The model under review builds one solid part; all positions refer to its coordinate system, in mm. Round coordinates to 2 decimals unless told otherwise and drop trailing zeros. Answer as a JSON object with one key per item and string values. Group by question number.
1. To check wall thickness, follow probe 1 along Y at (x, z) = (0, -487); probe 2 along Y at (x, z) = (-5, -238.5); probe 3 along Y at (x, z) = (-7.5, -543). State the ranges of each line that lie inside material, in increasing order. Write a range as [from, to].
2. Add section A-A on z = -559. Give the number of separate pieces and of enclosed holes in the cut face, and give its area (3 significant figures).
3. Clearance check with flat-ended pins moving along their axes: P1, Ø2.5, axis at x = 1.5, z = -398.5, coming from the +Y side; P2, Ø1.1, axis at x = 1.5, z = -214.5, coming from the -Y side. State where each tip first meets the part, or that it passes through.
```python
from build123d import *

# Parameters (mm, degrees)
SKETCH1_R           = 2.5
BOSS_EXTRUDE1_DEPTH = 550


with BuildPart() as part:
    # Sketch1 → Boss-Extrude1 (new body)
    with BuildSketch(Plane(origin=(0, 0, -600), x_dir=(-1, 0, 0), z_dir=(0, 0, -1))):
        with BuildLine():
            Line((10, -7), (10, 7))
            Line((10, 7), (8, 7))
            Line((8, 7), (8, 4))
            Line((8, 4), (7.060660172, 4))
            Line((7.060660172, 4), (4, 7.060660172))
            Line((4, 7.060660172), (4, 7.5))
            Line((4, 7.5), (3.750976592, 8.781114371))
            Line((3.750976592, 8.781114371), (3.933012702, 9.096410162))
            ThreePointArc((3.933012702, 9.096410162), (4, 9.346410162), (3.933012702, 9.596410162))
            Line((3.933012702, 9.596410162), (3.7, 10))
            Line((3.7, 10), (3.933012702, 10.403589838))
            ThreePointArc((3.933012702, 10.403589838), (3.982962913, 10.524180316), (4, 10.653589838))
            Line((4, 10.653589838), (4, 12.939339828))
            Line((4, 12.939339828), (7.060660172, 16))
            Line((7.060660172, 16), (8, 16))
            Line((8, 16), (8, 13))
            Line((8, 13), (10, 13))
            Line((10, 13), (10, 19))
            ThreePointArc((10, 19), (9.707106781, 19.707106781), (9, 20))
            Line((9, 20), (3, 20))
            Line((3, 20), (3, 18))
            Line((3, 18), (6, 18))
            Line((6, 18), (6, 17.060660172))
            Line((6, 17.060660172), (2.939339828, 14))
            Line((2.939339828, 14), (2.5, 14))
            Line((2.5, 14), (1.218885629, 13.750976592))
            Line((1.218885629, 13.750976592), (0.903589838, 13.933012702))
            ThreePointArc((0.903589838, 13.933012702), (0.653589838, 14), (0.403589838, 13.933012702))
            Line((0.403589838, 13.933012702), (0, 13.7))
            Line((0, 13.7), (-0.403589838, 13.933012702))
            ThreePointArc((-0.403589838, 13.933012702), (-0.524180316, 13.982962913), (-0.653589838, 14))
            Line((-0.653589838, 14), (-2.939339828, 14))
            Line((-2.939339828, 14), (-6, 17.060660172))
            Line((-6, 17.060660172), (-6, 18))
            Line((-6, 18), (-3, 18))
            Line((-3, 18), (-3, 20))
            Line((-3, 20), (-9, 20))
            ThreePointArc((-9, 20), (-9.707106781, 19.707106781), (-10, 19))
            Line((-10, 19), (-10, 13))
            Line((-10, 13), (-8, 13))
            Line((-8, 13), (-8, 16))
            Line((-8, 16), (-7.060660172, 16))
            Line((-7.060660172, 16), (-4, 12.939339828))
            Line((-4, 12.939339828), (-4, 12.5))
            Line((-4, 12.5), (-3.750976592, 11.218885629))
            Line((-3.750976592, 11.218885629), (-3.933012702, 10.903589838))
            ThreePointArc((-3.933012702, 10.903589838), (-4, 10.653589838), (-3.933012702, 10.403589838))
            Line((-3.933012702, 10.403589838), (-3.7, 10))
            Line((-3.7, 10), (-3.933012702, 9.596410162))
            ThreePointArc((-3.933012702, 9.596410162), (-3.982962913, 9.475819684), (-4, 9.346410162))
            Line((-4, 9.346410162), (-4, 7.060660172))
            Line((-4, 7.060660172), (-7.060660172, 4))
            Line((-7.060660172, 4), (-8, 4))
            Line((-8, 4), (-8, 7))
            Line((-8, 7), (-10, 7))
            Line((-10, 7), (-10, -7))
            Line((-10, -7), (-8, -7))
            Line((-8, -7), (-8, -4))
            Line((-8, -4), (-7.060660172, -4))
            Line((-7.060660172, -4), (-4, -7.060660172))
            Line((-4, -7.060660172), (-4, -9.346410162))
            ThreePointArc((-4, -9.346410162), (-3.982962913, -9.475819684), (-3.933012702, -9.596410162))
            Line((-3.933012702, -9.596410162), (-3.7, -10))
            Line((-3.7, -10), (-3.933012702, -10.403589838))
            ThreePointArc((-3.933012702, -10.403589838), (-4, -10.653589838), (-3.933012702, -10.903589838))
            Line((-3.933012702, -10.903589838), (-3.750976592, -11.218885629))
            Line((-3.750976592, -11.218885629), (-4, -12.5))
            Line((-4, -12.5), (-4, -12.939339828))
            Line((-4, -12.939339828), (-7.060660172, -16))
            Line((-7.060660172, -16), (-8, -16))
            Line((-8, -16), (-8, -13))
            Line((-8, -13), (-10, -13))
            Line((-10, -13), (-10, -19))
            ThreePointArc((-10, -19), (-9.707106781, -19.707106781), (-9, -20))
            Line((-9, -20), (-3, -20))
            Line((-3, -20), (-3, -18))
            Line((-3, -18), (-6, -18))
            Line((-6, -18), (-6, -17.060660172))
            Line((-6, -17.060660172), (-2.939339828, -14))
            Line((-2.939339828, -14), (-0.653589838, -14))
            ThreePointArc((-0.653589838, -14), (-0.524180316, -13.982962913), (-0.403589838, -13.933012702))
            Line((-0.403589838, -13.933012702), (0, -13.7))
            Line((0, -13.7), (0.403589839, -13.933012702))
            ThreePointArc((0.403589839, -13.933012702), (0.653589839, -14), (0.903589838, -13.933012702))
            Line((0.903589838, -13.933012702), (1.218885629, -13.750976592))
            Line((1.218885629, -13.750976592), (2.5, -14))
            Line((2.5, -14), (2.939339828, -14))
            Line((2.939339828, -14), (6, -17.060660172))
            Line((6, -17.060660172), (6, -18))
            Line((6, -18), (3, -18))
            Line((3, -18), (3, -20))
            Line((3, -20), (9, -20))
            ThreePointArc((9, -20), (9.707106781, -19.707106781), (10, -19))
            Line((10, -19), (10, -13))
            Line((10, -13), (8, -13))
            Line((8, -13), (8, -16))
            Line((8, -16), (7.060660172, -16))
            Line((7.060660172, -16), (4, -12.939339828))
            Line((4, -12.939339828), (4, -10.653589838))
            ThreePointArc((4, -10.653589838), (3.982962913, -10.524180316), (3.933012702, -10.403589838))
            Line((3.933012702, -10.403589838), (3.7, -10))
            Line((3.7, -10), (3.933012702, -9.596410162))
            ThreePointArc((3.933012702, -9.596410162), (4, -9.346410162), (3.933012702, -9.096410162))
            Line((3.933012702, -9.096410162), (3.750976592, -8.781114371))
            Line((3.750976592, -8.781114371), (4, -7.5))
            Line((4, -7.5), (4, -7.060660172))
            Line((4, -7.060660172), (7.060660172, -4))
            Line((7.060660172, -4), (8, -4))
            Line((8, -4), (8, -7))
            Line((8, -7), (10, -7))
        make_face()
        with Locations((0, -10)):
            Circle(SKETCH1_R, mode=Mode.SUBTRACT)
        with Locations((0, 10)):
            Circle(SKETCH1_R, mode=Mode.SUBTRACT)
        with BuildLine():
            Line((8, 1.7), (8, -1.7))
            ThreePointArc((8, -1.7), (7.912132034, -1.912132034), (7.7, -2))
            Line((7.7, -2), (7.063603897, -2))
            ThreePointArc((7.063603897, -2), (6.948798867, -2.02283614), (6.851471863, -2.087867966))
            Line((6.851471863, -2.087867966), (2.939339828, -6))
            Line((2.939339828, -6), (-2.939339828, -6))
            Line((-2.939339828, -6), (-6.851471863, -2.087867966))
            ThreePointArc((-6.851471863, -2.087867966), (-6.948798867, -2.02283614), (-7.063603897, -2))
            Line((-7.063603897, -2), (-7.7, -2))
            ThreePointArc((-7.7, -2), (-7.912132034, -1.912132034), (-8, -1.7))
            Line((-8, -1.7), (-8, 1.7))
            ThreePointArc((-8, 1.7), (-7.912132034, 1.912132034), (-7.7, 2))
            Line((-7.7, 2), (-7.063603897, 2))
            ThreePointArc((-7.063603897, 2), (-6.948798867, 2.02283614), (-6.851471863, 2.087867966))
            Line((-6.851471863, 2.087867966), (-2.939339828, 6))
            Line((-2.939339828, 6), (2.939339828, 6))
            Line((2.939339828, 6), (6.851471863, 2.087867966))
            ThreePointArc((6.851471863, 2.087867966), (6.948798867, 2.02283614), (7.063603897, 2))
            Line((7.063603897, 2), (7.7, 2))
            ThreePointArc((7.7, 2), (7.912132034, 1.912132034), (8, 1.7))
        make_face(mode=Mode.SUBTRACT)
    extrude(amount=-BOSS_EXTRUDE1_DEPTH)


solid = part.part
```
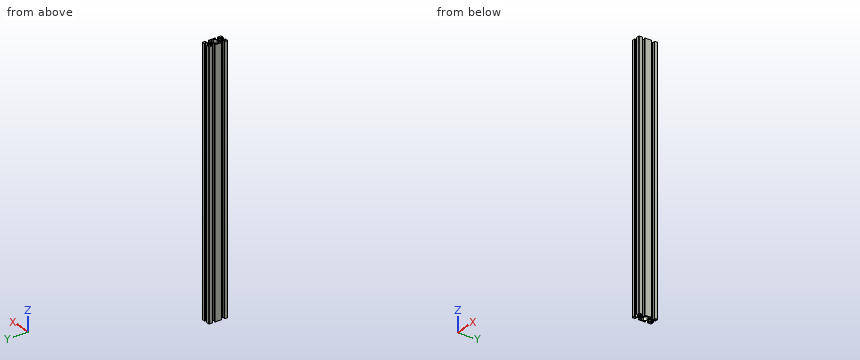
Recorded:
{
 "1": {"probe 1": "y = [-13.7, -12.5], [-7.5, -6], [6, 7.5], [12.5, 13.7]", "probe 2": "y = [-20, -18], [-16.06, -13.94], [-6.06, -3.94], [3.94, 6.06], [13.94, 16.06], [18, 20]", "probe 3": "y = [-20, -16], [-4, -2], [2, 4], [16, 20]"},
 "2": {"separate pieces": "1", "enclosed holes": "3", "area": "311 mm²"},
 "3": {"P1": "stops at y = 14", "P2": "stops at y = -14"}
}
